Read the model definition and answer for the solid it produces. Units are mm, in the model's axes. Face numbers are marked on the shaded views. A direction names the side the tool comes from. Coordinates: 2 decimals unless noted, no trailing zeros. Write each loop counter-clockwise with the first axis right and the second up, starting at its lowest first coordinate (ties: lowest second). Pieces come first, ordered by that corner, then holes. Notation, with made-up numbers: (-1, 11) -> (35, 11) arc R3 cw to (35, 15) -> close; hole circle Ø11 at (-17, 30.25). An arc over 180 degrees is marked (long way). Answer in a Markdown table with one row per item. Add a question column.
Item 1: Section A-A on y = 77.5 is taken. Write down the section's boundary in (x, z).
Item 2: For a pull along Y with two mould halves and no side action, classify the marked faces 1, 2, 3 and 4 as +Y half, -Y half, draft (parallel to the pull), parting line (faces both ways), or undercut.
Item 3: Straight lines are drawn through the part: line 1 (Y direction, x = 9.5, z = 2.25); line 2 (X direction, y = 90.5, z = 8); line 3 (Y direction, x = 8.5, z = 4.25). For each, find the intervals that lie inside material, in ascending order. Write a range as from..to.
Item 4: Section B-B on y = 90.5 is taken. Write down the section's boundary in (x, z), then the cut area to 3 significant figures.
Item 5: Section D-D on z = 5.25 is taken. Write down the section's boundary in (x, y), then the cut area to 3 significant figures.
Item 6: Which of the six approach directions +Z, -Z, +X, -X, +Y, -Y give full straight-line access (tool end or side, diameter ignored) to the marked faces 5 and 6?
Item 7: Section C-C on x = 9.5 is taken. Write down the section's boundary in (y, z), then the cut area to 3 significant figures.
Item 8: Given pin 1 Ø17.5 at (x, y) = (19.5, 75.5) entering from -Z; pin 2 Ø6 at (x, y) = (39, 35) entering from +Z; pin 3 Ø9 at (x, y) = (22.5, 77.5) entering from -Z, each flat-ended and moving along its own axis, determine where each tip first touches the part or whether it passes through.
```python
from build123d import *

# Parameters (mm, degrees)
SKETCH1_W           = 45
SKETCH1_H           = 100
BOSS_EXTRUDE1_DEPTH = 10
SKETCH3_R           = 7.5
SKETCH3_R_2         = 1.4
CUT_EXTRUDE1_DEPTH  = 10
SKETCH4_R           = 11
CUT_EXTRUDE2_DEPTH  = 2.2
SKETCH5_W           = 12
SKETCH5_H           = 0.8
CUT_EXTRUDE3_DEPTH  = 60
CHAMFER1_SIZE       = 2


with BuildPart() as part:
    # Sketch1 → Boss-Extrude1 (new body)
    with BuildSketch(Plane.XY):
        with Locations((22.5, 50)):
            Rectangle(SKETCH1_W, SKETCH1_H)
    extrude(amount=BOSS_EXTRUDE1_DEPTH)

    # Sketch3 → Cut-Extrude1 (cut)
    with BuildSketch(Plane.XY.offset(10)):
        with Locations((22.5, 77.5)):
            Circle(SKETCH3_R)
        with Locations((9.5, 90.5)):
            Circle(SKETCH3_R_2)
        with Locations((35.5, 90.5)):
            Circle(SKETCH3_R_2)
        with Locations((35.5, 64.5)):
            Circle(SKETCH3_R_2)
        with Locations((9.5, 64.5)):
            Circle(SKETCH3_R_2)
    extrude(amount=-CUT_EXTRUDE1_DEPTH, mode=Mode.SUBTRACT)

    # Sketch4 → Cut-Extrude2 (cut)
    with BuildSketch(Plane(origin=(0, 0, 0), x_dir=(-1, 0, 0), z_dir=(0, 0, -1))):
        with Locations((-22.5, 77.5)):
            Circle(SKETCH4_R)
    extrude(amount=-CUT_EXTRUDE2_DEPTH, mode=Mode.SUBTRACT)

    # Sketch5 → Cut-Extrude3 (cut)
    with BuildSketch(Plane.XZ):
        with Locations((6, 9.6)):
            Rectangle(SKETCH5_W, SKETCH5_H)
        with Locations((39, 9.6)):
            Rectangle(SKETCH5_W, SKETCH5_H)
    extrude(amount=-CUT_EXTRUDE3_DEPTH, mode=Mode.SUBTRACT)

    # Chamfer1
    chamfer1_edges = [part.edges().sort_by_distance(p)[0] for p in [
        (45, 0, 4.6),
        (0, 0, 4.6),
        (0, 100, 5),
        (45, 100, 5),
    ]]
    chamfer(chamfer1_edges, length=CHAMFER1_SIZE)


solid = part.part
```
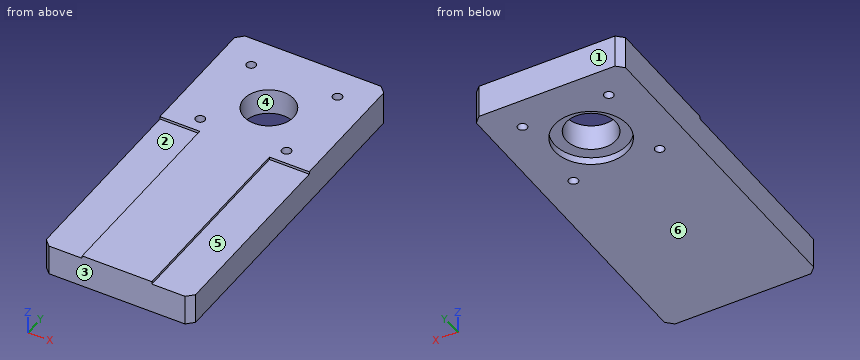
Results below:
| question | item | result |
|---|---|---|
| 1 | outline | (0, 0) -> (11.5, 0) -> (11.5, 2.2) -> (15, 2.2) -> (15, 10) -> (0, 10) -> close; (30, 2.2) -> (33.5, 2.2) -> (33.5, 0) -> (45, 0) -> (45, 10) -> (30, 10) -> close |
| 2 | face 1 | +Y half |
| 2 | face 2 | draft |
| 2 | face 3 | -Y half |
| 2 | face 4 | undercut |
| 3 | line 1 | y = 0..63.1, 65.9..89.1, 91.9..100 |
| 3 | line 2 | x = 0..8.1, 10.9..34.1, 36.9..45 |
| 3 | line 3 | y = 0..63.52, 65.48..89.52, 91.48..100 |
| 4 | outline | (0, 0) -> (8.1, 0) -> (8.1, 10) -> (0, 10) -> close; (10.9, 0) -> (34.1, 0) -> (34.1, 10) -> (10.9, 10) -> close; (36.9, 0) -> (45, 0) -> (45, 10) -> (36.9, 10) -> close |
| 4 | area | 394 mm2 |
| 5 | outline | (0, 2) -> (2, 0) -> (43, 0) -> (45, 2) -> (45, 98) -> (43, 100) -> (2, 100) -> (0, 98) -> close; hole circle Ø2.8 at (9.5, 64.5); hole circle Ø2.8 at (9.5, 90.5); hole circle Ø15 at (22.5, 77.5); hole circle Ø2.8 at (35.5, 64.5); hole circle Ø2.8 at (35.5, 90.5) |
| 5 | area | 4,290 mm2 |
| 6 | face 5 | +Z, +X, -Y |
| 6 | face 6 | -Z, +X, -X, +Y, -Y |
| 7 | outline | (0, 0) -> (63.1, 0) -> (63.1, 10) -> (60, 10) -> (60, 9.2) -> (0, 9.2) -> close; (65.9, 0) -> (89.1, 0) -> (89.1, 10) -> (65.9, 10) -> close; (91.9, 0) -> (100, 0) -> (100, 10) -> (91.9, 10) -> close |
| 7 | area | 896 mm2 |
| 8 | pin 1 | stops at z = 0 |
| 8 | pin 2 | stops at z = 9.2 |
| 8 | pin 3 | passes through |
